Read the model definition and answer for the solid it produces. Units are mm, in the model's axes. A direction names the side the tool comes from. Coordinates: 2 decimals unless noted, no trailing zeros. Order: outer loops, then holes, each group sorted by start corner. A loop starts at its lowest first (then second) coordinate and runs counter-clockwise, first axis right, second up. Notation, with made-up numbers: (61, 9) - (76, 9) arc R14 ccw to (76, 31) - close; hole circle Ø7 at (21.5, -1.5). An arc over 180 degrees is marked (long way). Write item = value, one per line.
from build123d import *

# Parameters (mm, degrees)
SKETCH1_W           = 90
SKETCH1_H           = 45
BOSS_EXTRUDE1_DEPTH = 117
SKETCH1_3_W         = 90
SKETCH1_3_H         = 36
BOSS_EXTRUDE2_DEPTH = 45
BOSS_EXTRUDE3_DEPTH = 27
CUT_EXTRUDE1_REACH  = 151.248
BOSS_EXTRUDE4_DEPTH = 9


with BuildPart() as part:
    # Sketch1 → Boss-Extrude1 (new body)
    with BuildSketch(Plane.XY):
        with Locations((0, 22.5)):
            Rectangle(SKETCH1_W, SKETCH1_H)
    extrude(amount=BOSS_EXTRUDE1_DEPTH)

    # Sketch1_3 → Boss-Extrude2 (add)
    with BuildSketch(Plane.XY):
        with Locations((0, 63)):
            Rectangle(SKETCH1_3_W, SKETCH1_3_H)
    extrude(amount=BOSS_EXTRUDE2_DEPTH)

    # Sketch1_4 → Boss-Extrude3 (add)
    with BuildSketch(Plane.XY):
        with BuildLine():
            ThreePointArc((-45, 81), (0, 126), (45, 81))
            Line((45, 81), (-45, 81))
        make_face()
        with BuildLine():
            Line((27, 90), (-27, 90))
            ThreePointArc((-27, 90), (0, 117), (27, 90))
        make_face(mode=Mode.SUBTRACT)
    extrude(amount=BOSS_EXTRUDE3_DEPTH)

    # Sketch5 → Cut-Extrude1 (cut, up to next)
    with BuildSketch(Plane(origin=(0, 45, 0), x_dir=(1, 0, 0), z_dir=(0, 1, 0)), mode=Mode.PRIVATE) as cut_extrude1_sk1:
        with BuildLine():
            Line((-27, -117), (27, -117))
            ThreePointArc((27, -117), (0, -90), (-27, -117))
        make_face()
    cut_extrude1_tool1 = extrude(cut_extrude1_sk1.sketch, amount=-CUT_EXTRUDE1_REACH, mode=Mode.PRIVATE) & part.part
    add(cut_extrude1_tool1.solids().sort_by_distance((0, 45, 105.540844))[0], mode=Mode.SUBTRACT)

    # Sketch7 → Boss-Extrude4 (add, symmetric)
    with BuildSketch(Plane(origin=(0, 0, 0), x_dir=(0, 0, -1), z_dir=(1, 0, 0))):
        Polygon((-45, 81), (-81, 45), (-45, 45), align=None)
    extrude(amount=BOSS_EXTRUDE4_DEPTH, both=True)


solid = part.part
1) Straight lines are drawn through the part: line 1 along Y through (x, z) = (-29.5, 108); line 2 along Y through (x, z) = (-25.5, 38.5). For each, find the intervals that lie inside material, in ascending order. Write a range as from..to.
Returned:
line_1 = 0..45
line_2 = 0..81
2) The part is cut by section C-C (z = 104.5). Determine the outline of the cut face in (x, y).
Returned:
outline = (-45, 0) - (-23.93, 0) - (-23.93, 45) - (-45, 45) - close; (23.93, 0) - (45, 0) - (45, 45) - (23.93, 45) - close
3) The part is cut by section A-A (x = 0). Determine the outline of the cut face in (y, z), and give its area (3 significant figures).
Returned:
outline = (0, 0) - (90, 0) - (90, 27) - (81, 27) - (81, 45) - (45, 81) - (45, 90) - (0, 90) - close; (117, 0) - (126, 0) - (126, 27) - (117, 27) - close
area = 6,800 mm^2
4) The part is cut by section B-B (y = 115). Determine the outline of the cut face in (x, z).
Returned:
outline = (-29.48, 0) - (-10.2, 0) - (-10.2, 27) - (-29.48, 27) - close; (10.2, 0) - (29.48, 0) - (29.48, 27) - (10.2, 27) - close
5) Flat-ended cylindrical pins translate along their axes: pin 1 Ø5 at (y, z) = (48, 95) entering from -X; pin 2 Ø4 at (x, z) = (-8, 38.5) entering from +Y; pin 3 Ø1.5 at (x, y) = (-17.5, 28.5) entering from -Z; pin 4 Ø21.5 at (x, z) = (7.5, 18.5) entering from +Y. Find the tip coordinate at first contact, or state that the pin passes through.
Returned:
pin_1 = through
pin_2 = 81
pin_3 = 0
pin_4 = 126
6) For faces 1 (the face through (9, 55, 55)), 2 (the face through (-1, 81, 36)), 3 (the face through (-0.594, 116.993, 13.311)), 4 (the face through (9.4, 45, 80.5)), 5 (the face through (-9, 55, 55)), determine the directions among +Z, -Z, +X, -X, +Y, -Y from which every point of the face is accessible in a straight line to the end or side of a thin tool.
Returned:
face_1 = +Z, +X, +Y
face_2 = +Z, +X, -X, +Y
face_3 = +Z, -Z
face_4 = +Z, +Y
face_5 = +Z, -X, +Y
7) Determine the mould class of faces 6 (the face through (0, 90, 13)), 7 (the face through (-0.99, 125.99, 13.31)), 8 (the face through (0.594, 22.815, 90.007)) for opening direction Y: pulls with the +Y half, pulls with the -Y half, needs draft (parallel to the pull), parting line crosses it, or undercut.
Returned:
face_6 = undercut
face_7 = pulls with the +Y half
face_8 = needs draft
8) The part is cut by section D-D (y = 62.5). Determine the outline of the cut face in (x, z), and give its area (3 significant figures).
Returned:
outline = (-45, 0) - (45, 0) - (45, 45) - (9, 45) - (9, 63.5) - (-9, 63.5) - (-9, 45) - (-45, 45) - close
area = 4,380 mm^2
